For this review, take the finished solid that the model builds, in its own axes (mm). Round coordinates to 2 decimals unless told otherwise and drop trailing zeros. Loops run counter-clockwise (first coordinate to the right, second up) from the corner with the lowest first, then second, coordinate; pieces in that order, holes last. Notation, with made-up numbers: (34, -10) -> (64, -10) arc R9 cw to (64, 6) -> close; hole circle Ø3 at (-27.5, -17). An arc over 180 degrees is marked (long way). One line per question, with ' | ' between items. Start each with the question number.
1. Draft analysis for pull direction X (two halves, no side actions). For faces 1 (the face through (-19.6, 81.51, 381.19)), 2 (the face through (-1.186, 75.915, 407.483)), 3 (the face through (93.32, 85.44, 359.22)), state which applies: pulls with the +X half, pulls with the -X half, needs draft (parallel to the pull), parting line crosses it, or undercut.
2. For pin 1 Ø4 at (x, y) = (69.5, 80) entering from +Z; pin 2 Ø10 at (y, z) = (81.5, 402) entering from +X; pin 3 Ø1.5 at (x, z) = (-9, 365) entering from +Y; pin 4 Ø6 at (x, z) = (66.5, 402.5) entering from -Y, all flat-tipped, find the tip position at first contact; note any pin that passes through.
3. Consider section B-B (z = 359.5). Write out the cut boundary in (x, y).
4. Consider section A-A (x = 43.5). Write out the cut boundary in (y, z).
5. Wall thickness on line 1 along X through (y, z) = (77, 391.5) (3 decimals); line 2 along X through (y, z) = (83.5, 368); line 3 along Y through (x, z) = (2.5, 357.5): over which ranges is each line inside the solid? List them lowest first.
```python
from build123d import *

# Parameters (mm, degrees)
BOSS_EXTRUDE1_DEPTH = 6.35
SKETCH4_R           = 1.190625
CUT_EXTRUDE2_DEPTH  = 398.434844364


with BuildPart() as part:
    # Sketch2 → Boss-Extrude1 (new body)
    with BuildSketch(Plane(origin=(0.683346332, 150.385179261, 31.029771586), x_dir=(-0.9999900978792948, 0.004358374370466655, 0.0008992864979534574), z_dir=(0.004450184643196504, 0.979359636230067, 0.20207646765507412))):
        Polygon((-88.422343932, 329.663853712), (90.808907549, 329.663853712), (97.754590844, 340.296232729), (97.754590844, 383.735739743), (-96.711451797, 383.735739743), (-96.711451797, 339.285739743), align=None)
    extrude(amount=BOSS_EXTRUDE1_DEPTH)

    # Sketch4 → Cut-Extrude2 (cut, through all)
    with BuildSketch(Plane(origin=(0.711605005, 156.604112951, 32.312957155), x_dir=(0.9999900978792948, -0.0043583743704666555, -0.0008992864979534572), z_dir=(0.004450184643196505, 0.9793596362300672, 0.2020764676550741))):
        with Locations(Location((17.856718191, -355.665986236, 0), (0, 0, 270))):
            Circle(SKETCH4_R)
        with Locations(Location((17.856718191, -368.365986236, 0), (0, 0, 90))):
            Circle(SKETCH4_R)
        with Locations(Location((-20.243281809, -368.365986236, 0), (0, 0, 270))):
            Circle(SKETCH4_R)
        with Locations(Location((-20.243281809, -355.665986236, 0), (0, 0, 90))):
            Circle(SKETCH4_R)
    extrude(amount=-CUT_EXTRUDE2_DEPTH, mode=Mode.SUBTRACT)


solid = part.part
```
Answer block:
1) face 1: undercut | face 2: needs draft | face 3: pulls with the +X half
2) pin 1: stops at z = 408.07 | pin 2: stops at x = 97.42 | pin 3: stops at y = 88.16 | pin 4: stops at y = 72.82
3) outline: (-93.81, 83.04) -> (94.11, 82.19) -> (93.01, 88.67) -> (-92.92, 89.52) -> close
4) outline: (72.65, 406.81) -> (83.58, 353.85) -> (89.8, 355.14) -> (78.87, 408.09) -> close
5) line 1: x = -97.068 to -20.635, -18.477 to 17.465, 19.624 to 97.4 | line 2: x = -97.06 to 97.41 | line 3: y = 83.01 to 89.5
